Work out the finished part from the listing and answer in its coordinate system (mm). Face numbers are marked on the shaded views. A direction names the side the tool comes from. Coordinates: 2 decimals unless noted, no trailing zeros. Loops run counter-clockwise (first coordinate to the right, second up) from the corner with the lowest first, then second, coordinate; pieces in that order, holes last. Notation, with made-up numbers: (47, 54.25) -> (76, 54.25) arc R22 ccw to (76, 93.25) -> close; hole circle Ø2 at (56, 27). An arc over 180 degrees is marked (long way). Use a Markdown table: item, result.
from build123d import *

# Parameters (mm, degrees)
SKETCH064_R     = 2.3
PAD044_DEPTH    = 3
PAD045_DEPTH    = 1.5
SKETCH066_W     = 3
SKETCH066_H     = 1
POCKET013_DEPTH = 0.6
CHAMFER007_SIZE = 0.1


with BuildPart() as part:
    # Sketch064 → Pad044 (new body)
    with BuildSketch(Plane.XY):
        Circle(SKETCH064_R)
    extrude(amount=PAD044_DEPTH)

    # Sketch065 (on Face3 of Pad044) → Pad045 (join)
    with BuildSketch(Plane.XY.offset(3)):
        with BuildLine():
            Line((0.425, 2.767558), (0.425, 3.617558))
            Line((0.425, 3.617558), (-0.425, 3.617558))
            Line((-0.425, 3.617558), (-0.425, 2.767558))
            ThreePointArc((-0.425, 2.767558), (0, -2.8), (0.425, 2.767558))
        make_face()
    extrude(amount=PAD045_DEPTH)

    # Sketch066 → Pocket013 (cut)
    with BuildSketch(Plane.XY):
        Rectangle(SKETCH066_W, SKETCH066_H)
    extrude(amount=POCKET013_DEPTH, mode=Mode.SUBTRACT)

    # Chamfer007
    chamfer007_edges = [part.edges().sort_by_distance(p)[0] for p in [
        (0, -0.5, 0),
        (-2.3, 0, 0),
        (-1.5, 0, 0),
        (0, 0.5, 0),
        (1.5, 0, 0),
    ]]
    chamfer(chamfer007_edges, length=CHAMFER007_SIZE)


with BuildPart() as part_1:
    # Body019 placement: moved
    add(part.part.moved(Location((63.6, 11.5, -1.5))))


solid = part_1.part
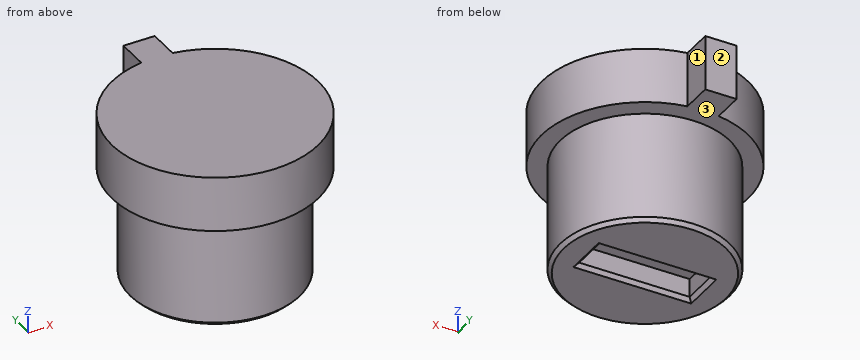
Q1. Section A-A on x = 63.6 is taken. Determine the outline of the cut face in (y, z).
Solved:
| item | result |
|---|---|
| outline | (8.7, 1.5) -> (9.2, 1.5) -> (9.2, -1.4) -> (9.3, -1.5) -> (10.9, -1.5) -> (11, -1.4) -> (11, -0.9) -> (12, -0.9) -> (12, -1.4) -> (12.1, -1.5) -> (13.7, -1.5) -> (13.8, -1.4) -> (13.8, 1.5) -> (15.12, 1.5) -> (15.12, 3) -> (8.7, 3) -> close |
Q2. Section C-C on z = 0.15 is taken. Determine the outline of the cut face in (x, y), and give its area (3 significant figures).
Solved:
| item | result |
|---|---|
| outline | circle Ø4.6 at (63.6, 11.5) |
| area | 16.6 mm² |
Q3. Given pin 1 Ø1.5 at (y, z) = (11.5, -0.5) entering from -X; pin 2 Ø1.1 at (x, y) = (63.5, 11.5) entering from -Z; pin 3 Ø1.5 at (x, z) = (65, -1) entering from -Y, each flat-ended and moving along its own axis, determine where each tip first touches the part or whether it passes through.
Solved:
| item | result |
|---|---|
| pin 1 | x = 61.3 |
| pin 2 | z = -1.45 |
| pin 3 | y = 9.29 |
Q4. Consider line 1 (Y direction, x = 63.5, z = 2.05); line 2 (Z direction, x = 61.2, y = 10.75); line 3 (Y direction, x = 62.8, z = -0.4). Determine where each line is inside the solid, lowest interval first. Write a range as [from, to].
Solved:
| item | result |
|---|---|
| line 1 | [8.7, 15.12] |
| line 2 | [1.5, 3] |
| line 3 | [9.34, 13.66] |
Q5. Section D-D on z = 1.9 is taken. Determine the outline of the cut face in (x, y) (3 decimals), and give its area (3 significant figures).
Solved:
| item | result |
|---|---|
| outline | (63.175, 14.268) arc R2.8 ccw (long way) to (64.025, 14.268) -> (64.025, 15.118) -> (63.175, 15.118) -> close |
| area | 25.3 mm² |
Q6. For the marked faces 1, 2 and 3, determine the directions among +Z, -Z, +X, -X, +Y, -Y from which every point of the face is accessible in a straight line to the end or side of a thin tool.
Solved:
| item | result |
|---|---|
| face 1 | +Z, -Z, +X, +Y |
| face 2 | +Z, -Z, +X, -X, +Y |
| face 3 | -Z |
Q7. Section B-B on y = 11.5 is taken. Determine the outline of the cut face in (x, z), and give its area (3 significant figures).
Solved:
| item | result |
|---|---|
| outline | (60.8, 1.5) -> (61.3, 1.5) -> (61.3, -1.4) -> (61.4, -1.5) -> (62, -1.5) -> (62.1, -1.4) -> (62.1, -0.9) -> (65.1, -0.9) -> (65.1, -1.4) -> (65.2, -1.5) -> (65.8, -1.5) -> (65.9, -1.4) -> (65.9, 1.5) -> (66.4, 1.5) -> (66.4, 3) -> (60.8, 3) -> close |
| area | 20.4 mm² |
